Study the drawing (mm; zero at the part's minimum x, y, z) and answer. Give positions to 0.01 mm unless a question says otherwise; leave off trailing zeros. Order: outer loops, then holes, each group sorted by start corner. A loop starts at its lowest first (then second) coordinate and runs counter-clockwise, first axis right, second up.
Item 1: Find the intervals of material crossed by line 1 along X through (y, z) = (31.75, 3); line 2 along Z through (x, y) = (19.05, 35.5); line 3 along Y through (x, z) = (19.05, 3.25), in increasing order.
Item 2: The mould has two halves that part along X. Classify the marked faces 1, 2 and 3: +X half, -X half, draft (parallel to the pull), parting line (faces both ways), or undercut.
Item 3: A cutting plane is placed at A-A (y = 31.75). Write down the section's boundary in (x, z), plus the area to 3 significant figures.
Item 4: A cutting plane is placed at C-C (z = 6.35). Write down the section's boundary in (x, y).
Item 5: Given pin 1 Ø6 at (x, z) = (19.05, 6.35) entering from -Y; pin 2 Ø4 at (x, y) = (6.35, 31.75) entering from +Z, each flat-ended and moving along its own axis, determine where each tip first touches the part or whether it passes through.
Item 6: A cutting plane is placed at B-B (x = 6.35). Write down the section's boundary in (y, z).
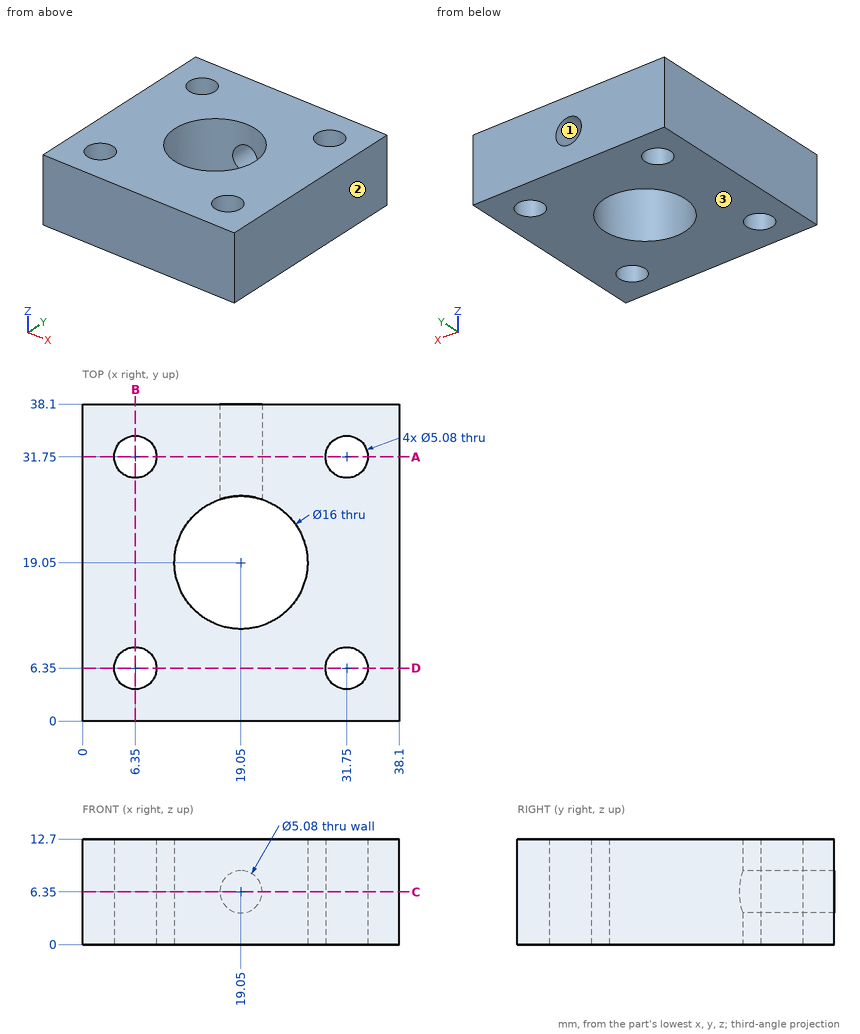
Response values:
1. line 1: x = 0 to 3.81, 8.89 to 29.21, 34.29 to 38.1
1. line 2: z = 0 to 3.81, 8.89 to 12.7
1. line 3: y = 0 to 11.05, 27.05 to 38.1
2. face 1: undercut
2. face 2: +X half
2. face 3: draft
3. outline: (0, 0) - (3.81, 0) - (3.81, 12.7) - (0, 12.7) - close; (8.89, 0) - (29.21, 0) - (29.21, 12.7) - (8.89, 12.7) - close; (34.29, 0) - (38.1, 0) - (38.1, 12.7) - (34.29, 12.7) - close; hole circle Ø5.08 at (19.05, 6.35)
3. area: 335 mm2
4. outline: (0, 0) - (38.1, 0) - (38.1, 38.1) - (21.59, 38.1) - (21.59, 26.64) arc R8 cw (long way) to (16.51, 26.64) - (16.51, 38.1) - (0, 38.1) - close; hole circle Ø5.08 at (6.35, 6.35); hole circle Ø5.08 at (6.35, 31.75); hole circle Ø5.08 at (31.75, 6.35); hole circle Ø5.08 at (31.75, 31.75)
5. pin 1: stops at y = 0
5. pin 2: passes through
6. outline: (0, 0) - (3.81, 0) - (3.81, 12.7) - (0, 12.7) - close; (8.89, 0) - (29.21, 0) - (29.21, 12.7) - (8.89, 12.7) - close; (34.29, 0) - (38.1, 0) - (38.1, 12.7) - (34.29, 12.7) - close
